Check sheet for the modelled part. Datum: model origin and axes. Units: mm. Face numbers are marked on the shaded views. A direction names the side the tool comes from. Give positions to 0.01 mm unless a question says otherwise; leave off trailing zeros. Loops run counter-clockwise (first coordinate to the right, second up) from the corner with the lowest first, then second, coordinate; pieces in that order, holes last. Notation, with made-up numbers: (16.5, 1.25) - (72.5, 1.25) arc R29 cw to (72.5, 25.25) - close; hole circle Ø2 at (-15, 75). An arc over 180 degrees is marked (long way). Use CSV: the item, a comma, the result in double quotes.
from build123d import *

# Parameters (mm, degrees)
SKETCH2_W            = 120
SKETCH2_H            = 120
BOSS_EXTRUDE1_DEPTH  = 50
SKETCH3_R            = 35
BOSS_EXTRUDE2_DEPTH  = 25
SKETCH4_R            = 25
CUT_EXTRUDE1_DEPTH   = 186.539753153
FILLET1_R            = 5
FILLET2_R            = 1.5
SHELL1_OUTLINE_W     = 116
SHELL1_OUTLINE_H     = 116
SHELL1_OUTLINE_R     = 27
SHELL1_DEPTH         = 45
SHELL1_2_OUTLINE_R   = 33
SHELL1_2_OUTLINE_R_2 = 27
SHELL1_2_DEPTH       = 73
SHELL1_START         = -118
SHELL1_3_DEPTH       = 116
SHELL1_START_2       = 1
SHELL1_4_DEPTH       = 118
SHELL1_START_3       = 45
SHELL1_5_OUTLINE_R   = 27
SHELL1_5_OUTLINE_R_2 = 25
SHELL1_5_DEPTH       = 3


with BuildPart() as part:
    # Sketch2 → Boss-Extrude1 (new body)
    with BuildSketch(Plane.XY):
        with Locations((-60, 60)):
            Rectangle(SKETCH2_W, SKETCH2_H)
    extrude(amount=BOSS_EXTRUDE1_DEPTH)

    # Sketch3 → Boss-Extrude2 (add)
    with BuildSketch(Plane.XY.offset(50)):
        with Locations((-60, 60)):
            Circle(SKETCH3_R)
    extrude(amount=BOSS_EXTRUDE2_DEPTH)

    # Sketch4 → Cut-Extrude1 (cut, through all)
    with BuildSketch(Plane.XY.offset(75)):
        with Locations((-60, 60)):
            Circle(SKETCH4_R)
    extrude(amount=-CUT_EXTRUDE1_DEPTH, mode=Mode.SUBTRACT)

    # Fillet1
    fillet1_edges = [part.edges().sort_by_distance(p)[0] for p in [
        (-120, 60, 50),
        (-60, 0, 50),
        (0, 60, 50),
        (-60, 120, 50),
    ]]
    fillet(fillet1_edges, radius=FILLET1_R)

    # Fillet2
    fillet2_edges = [part.edges().sort_by_distance(p)[0] for p in [
        (-95, 60, 75),
        (-85, 60, 75),
    ]]
    fillet(fillet2_edges, radius=FILLET2_R)

    # Shell1: read off the stored shape, not the designer's step
    # Shell1 outline → Shell1 (cut)
    with BuildSketch(Plane.XY):
        with Locations((-60, 60)):
            Rectangle(SHELL1_OUTLINE_W, SHELL1_OUTLINE_H)
        with Locations((-60, 60)):
            Circle(SHELL1_OUTLINE_R, mode=Mode.SUBTRACT)
    extrude(amount=SHELL1_DEPTH, mode=Mode.SUBTRACT)

    # Shell1 2 outline → Shell1 2 (cut)
    with BuildSketch(Plane.XY):
        with Locations((-60, 60)):
            Circle(SHELL1_2_OUTLINE_R)
        with Locations((-60, 60)):
            Circle(SHELL1_2_OUTLINE_R_2, mode=Mode.SUBTRACT)
    extrude(amount=SHELL1_2_DEPTH, mode=Mode.SUBTRACT)

    # Shell1 3 outline → Shell1 3 (cut)
    with BuildSketch(Plane.YZ.offset(SHELL1_START)):
        with BuildLine():
            ThreePointArc((118, 45), (117.121320344, 47.121320344), (115, 48))
            Line((115, 48), (5, 48))
            ThreePointArc((5, 48), (2.878679656, 47.121320344), (2, 45))
            Line((2, 45), (118, 45))
        make_face()
    extrude(amount=SHELL1_3_DEPTH, mode=Mode.SUBTRACT)

    # Shell1 4 outline → Shell1 4 (add)
    with BuildSketch(Plane(origin=(0, 0, 0), x_dir=(1, 0, 0), z_dir=(0, 1, 0)).offset(SHELL1_START_2)):
        with BuildLine():
            ThreePointArc((-2, -45), (-2.878679656, -47.121320344), (-5, -48))
            Line((-5, -48), (-2, -48))
            Line((-2, -48), (-2, -45))
        make_face()
        with BuildLine():
            ThreePointArc((-115, -48), (-117.121320344, -47.121320344), (-118, -45))
            Line((-118, -45), (-118, -48))
            Line((-118, -48), (-115, -48))
        make_face()
    extrude(amount=SHELL1_4_DEPTH)

    # Shell1 5 outline → Shell1 5 (add)
    with BuildSketch(Plane.XY.offset(SHELL1_START_3)):
        with Locations((-60, 60)):
            Circle(SHELL1_5_OUTLINE_R)
        with Locations((-60, 60)):
            Circle(SHELL1_5_OUTLINE_R_2, mode=Mode.SUBTRACT)
    extrude(amount=SHELL1_5_DEPTH)


solid = part.part
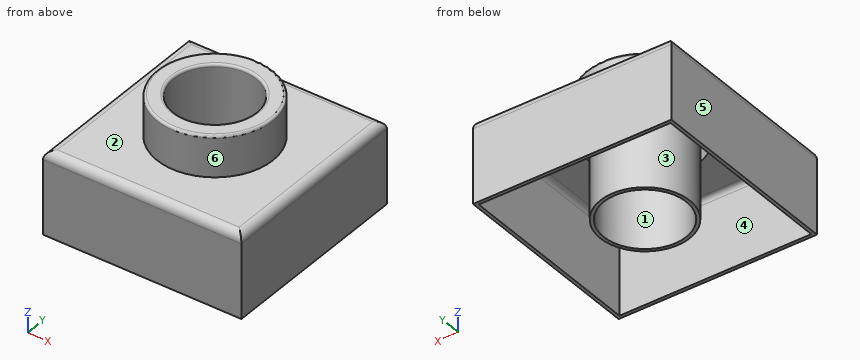
1. Sectioned sample at D-D, the plane y = 96.5. Record the boundary of the cut face in (x, z).
Completed:
outline,"(-120, 0) - (-118, 0) - (-118, 45) arc R3 cw to (-115, 48) - (-5, 48) arc R3 cw to (-2, 45) - (-2, 0) - (0, 0) - (0, 45) arc R5 ccw to (-5, 50) - (-115, 50) arc R5 ccw to (-120, 45) - close"
2. Set-up check for the marked faces 1, 2 and 3: record each of +Z, -Z, +X, -X, +Y, -Y from which the full face is reachable in a straight line by a thin tool's end or side.
Completed:
face 1,"+Z, -Z"
face 2,"+Z"
face 3,"-Z"
3. Sectioned sample at A-A, the plane z = 18. Record the boundary of the cut face in (x, y).
Completed:
outline,"(-120, 0) - (0, 0) - (0, 120) - (-120, 120) - close; circle Ø54 at (-60, 60); hole (-118, 2) - (-2, 2) - (-2, 118) - (-118, 118) - close; hole circle Ø50 at (-60, 60)"
4. Release check for a two-part mould opening along Y. For the marked faces 4, 5 and 6 record: released by +Y, released by -Y, zero draft, split by the parting line, or undercut.
Completed:
face 4,"undercut"
face 5,"zero draft"
face 6,"split by the parting line"
5. Go/stop test with flat-tipped pins: pin 1 Ø3 at (x, z) = (-96.5, 17) entering from -Y; pin 2 Ø3 at (y, z) = (68, 63) entering from +X; pin 3 Ø3 at (x, y) = (-43, 17) entering from -Z; pin 4 Ø4 at (x, y) = (-93, 46) entering from +Z. Record where each tip stops, or that it passes through.
Completed:
pin 1,"stops at y = 0"
pin 2,"stops at x = -25.61"
pin 3,"stops at z = 48"
pin 4,"stops at z = 74.96"
6. Scan lines: line 1 along Y through (x, z) = (-60, 54); line 2 along Y through (x, z) = (-60, 22); line 3 along Y through (x, z) = (-17.5, 8). Record each from-to range of solid material in increasing order.
Completed:
line 1,"y = 25 to 27, 33 to 35, 85 to 87, 93 to 95"
line 2,"y = 0 to 2, 33 to 35, 85 to 87, 118 to 120"
line 3,"y = 0 to 2, 118 to 120"
